Read the model definition and answer for the solid it produces. Units are mm, in the model's axes. A direction names the side the tool comes from. Coordinates: 2 decimals unless noted, no trailing zeros. Order: outer loops, then holes, each group sorted by start corner. A loop starts at its lowest first (then second) coordinate and runs counter-clockwise, first axis right, second up. Notation, with made-up numbers: (-4, 15) - (38, 15) arc R18 cw to (38, 42) - close; hole circle Ø9 at (-0.75, 27.5). An arc over 180 degrees is marked (long way). Write item = value, one per line.
from build123d import *

# Parameters (mm, degrees)
SKETCH1_W              = 116.84
SKETCH1_H              = 103.134084814
SKETCH1_R              = 3.15
BOSS_EXTRUDE1_DEPTH    = 5
SKETCH12_W             = 85
SKETCH12_H             = 23.975046692
BOSS_EXTRUDE15_DEPTH   = 5
SKETCH17_W             = 50
SKETCH17_H             = 50
BOSS_EXTRUDE18_DEPTH   = 6
SKETCH10_W             = 39.5
SKETCH10_H             = 39.5
BOSS_EXTRUDE19_DEPTH   = 25
SKETCH19_W             = 55
SKETCH19_H             = 55
BOSS_EXTRUDE20_DEPTH   = 11
SKETCH20_R             = 2.25
BOSS_EXTRUDE22_DEPTH   = 25
BOSS_EXTRUDE22_2_DEPTH = 25
BOSS_EXTRUDE22_3_DEPTH = 25
BOSS_EXTRUDE22_4_DEPTH = 25
SKETCH21_W             = 24.5
SKETCH21_H             = 21.5
BOSS_EXTRUDE23_DEPTH   = 4
SKETCH21_W_2           = 21.5
SKETCH21_H_2           = 24.5
BOSS_EXTRUDE23_2_DEPTH = 4
BOSS_EXTRUDE23_3_DEPTH = 4
BOSS_EXTRUDE23_4_DEPTH = 4
SKETCH25_R             = 4
BOSS_EXTRUDE24_DEPTH   = 3.25
BOSS_EXTRUDE24_2_DEPTH = 3.25
BOSS_EXTRUDE24_3_DEPTH = 3.25
BOSS_EXTRUDE24_4_DEPTH = 3.25


with BuildPart() as part:
    # Sketch1 → Boss-Extrude1 (new body)
    with BuildSketch(Plane(origin=(0, 0, 0), x_dir=(1, 0, 0), z_dir=(0, 1, 0))):
        with Locations((0, 1.415042407)):
            Rectangle(SKETCH1_W, SKETCH1_H)
        with Locations((-50.8, 46.711)):
            Circle(SKETCH1_R, mode=Mode.SUBTRACT)
        with Locations((50.8, -42.532)):
            Circle(SKETCH1_R, mode=Mode.SUBTRACT)
        with Locations((-50.8, -42.532)):
            Circle(SKETCH1_R, mode=Mode.SUBTRACT)
        with Locations((50.8, 46.711)):
            Circle(SKETCH1_R, mode=Mode.SUBTRACT)
    extrude(amount=-BOSS_EXTRUDE1_DEPTH)


with BuildPart() as body_2:
    # Sketch12 → Boss-Extrude15 (new body)
    with BuildSketch(Plane(origin=(0, 0, 0), x_dir=(1, 0, 0), z_dir=(0, 1, 0))):
        with Locations((0, 58)):
            Rectangle(SKETCH12_W, SKETCH12_H)
    extrude(amount=BOSS_EXTRUDE15_DEPTH)


with BuildPart() as body_3:
    # Sketch17 → Boss-Extrude18 (new body)
    with BuildSketch(Plane(origin=(0, 0, 0), x_dir=(1, 0, 0), z_dir=(0, 1, 0))):
        Rectangle(SKETCH17_W, SKETCH17_H)
    extrude(amount=-BOSS_EXTRUDE18_DEPTH)


with BuildPart() as body_4:
    # Sketch10 → Boss-Extrude19 (new body, symmetric)
    with BuildSketch(Plane(origin=(0, 0, 0), x_dir=(1, 0, 0), z_dir=(0, 1, 0))):
        Rectangle(SKETCH10_W, SKETCH10_H)
    extrude(amount=BOSS_EXTRUDE19_DEPTH, both=True)


with BuildPart() as body_5:
    # Sketch19 → Boss-Extrude20 (new body)
    with BuildSketch(Plane(origin=(0, 0, 0), x_dir=(1, 0, 0), z_dir=(0, 1, 0))):
        Rectangle(SKETCH19_W, SKETCH19_H)
    extrude(amount=-BOSS_EXTRUDE20_DEPTH)


with BuildPart() as part_1:
    add(part.part)

    # Combine1: cut body 2
    add(body_2.part, mode=Mode.SUBTRACT)


with BuildPart() as body_3_1:
    # Body-Move/Copy4: moved
    add(body_3.part.moved(Location((0, -6, 0))))


with BuildPart() as body_5_1:
    add(body_5.part)

    # Combine4: cut body 3
    add(body_3_1.part, mode=Mode.SUBTRACT)

    # Combine7: union part
    add(part_1.part)

    # Combine8: cut body 4
    add(body_4.part, mode=Mode.SUBTRACT)


with BuildPart() as body_2_2:
    # Sketch20 → Boss-Extrude22 (new body, symmetric)
    with BuildSketch(Plane(origin=(0, 0, 0), x_dir=(1, 0, 0), z_dir=(0, 1, 0))):
        with Locations((27.5, 27.5)):
            Circle(SKETCH20_R)
    extrude(amount=BOSS_EXTRUDE22_DEPTH, both=True)


with BuildPart() as body_3_2:
    # Sketch20 → Boss-Extrude22 2 (new body, symmetric)
    with BuildSketch(Plane(origin=(0, 0, 0), x_dir=(1, 0, 0), z_dir=(0, 1, 0))):
        with Locations((27.5, -27.5)):
            Circle(SKETCH20_R)
    extrude(amount=BOSS_EXTRUDE22_2_DEPTH, both=True)


with BuildPart() as body_4_2:
    # Sketch20 → Boss-Extrude22 3 (new body, symmetric)
    with BuildSketch(Plane(origin=(0, 0, 0), x_dir=(1, 0, 0), z_dir=(0, 1, 0))):
        with Locations((-27.5, -27.5)):
            Circle(SKETCH20_R)
    extrude(amount=BOSS_EXTRUDE22_3_DEPTH, both=True)


with BuildPart() as body_5_2:
    # Sketch20 → Boss-Extrude22 4 (new body, symmetric)
    with BuildSketch(Plane(origin=(0, 0, 0), x_dir=(1, 0, 0), z_dir=(0, 1, 0))):
        with Locations((-27.5, 27.5)):
            Circle(SKETCH20_R)
    extrude(amount=BOSS_EXTRUDE22_4_DEPTH, both=True)


with BuildPart() as body_5_3:
    add(body_5_1.part)

    # Combine9: cut body 4 2, body 3 2, body 2 2, body 5 2
    add(body_4_2.part, mode=Mode.SUBTRACT)
    add(body_3_2.part, mode=Mode.SUBTRACT)
    add(body_2_2.part, mode=Mode.SUBTRACT)
    add(body_5_2.part, mode=Mode.SUBTRACT)


with BuildPart() as body_2_3:
    # Sketch21 → Boss-Extrude23 (new body)
    with BuildSketch(Plane(origin=(0, 0, 0), x_dir=(1, 0, 0), z_dir=(0, 1, 0))):
        with Locations((0, 31.5)):
            Rectangle(SKETCH21_W, SKETCH21_H)
    extrude(amount=-BOSS_EXTRUDE23_DEPTH)


with BuildPart() as body_3_3:
    # Sketch21 → Boss-Extrude23 2 (new body)
    with BuildSketch(Plane(origin=(0, 0, 0), x_dir=(1, 0, 0), z_dir=(0, 1, 0))):
        with Locations((31.5, 0)):
            Rectangle(SKETCH21_W_2, SKETCH21_H_2)
    extrude(amount=-BOSS_EXTRUDE23_2_DEPTH)


with BuildPart() as body_4_3:
    # Sketch21 → Boss-Extrude23 3 (new body)
    with BuildSketch(Plane(origin=(0, 0, 0), x_dir=(1, 0, 0), z_dir=(0, 1, 0))):
        with Locations((-31.5, 0)):
            Rectangle(SKETCH21_W_2, SKETCH21_H_2)
    extrude(amount=-BOSS_EXTRUDE23_3_DEPTH)


with BuildPart() as body_5_3_1:
    # Sketch21 → Boss-Extrude23 4 (new body)
    with BuildSketch(Plane(origin=(0, 0, 0), x_dir=(1, 0, 0), z_dir=(0, 1, 0))):
        with Locations((0, -31.5)):
            Rectangle(SKETCH21_W, SKETCH21_H)
    extrude(amount=-BOSS_EXTRUDE23_4_DEPTH)


with BuildPart() as body_5_4:
    add(body_5_3.part)

    # Combine10: cut body 3 3, body 2 3, body 5 3, body 4 3
    add(body_3_3.part, mode=Mode.SUBTRACT)
    add(body_2_3.part, mode=Mode.SUBTRACT)
    add(body_5_3_1.part, mode=Mode.SUBTRACT)
    add(body_4_3.part, mode=Mode.SUBTRACT)


with BuildPart() as body_2_4:
    # Sketch25 → Boss-Extrude24 (new body)
    with BuildSketch(Plane(origin=(0, 0, 0), x_dir=(1, 0, 0), z_dir=(0, 1, 0))):
        with Locations((27.5, 27.5)):
            Circle(SKETCH25_R)
    extrude(amount=-BOSS_EXTRUDE24_DEPTH)


with BuildPart() as body_3_4:
    # Sketch25 → Boss-Extrude24 2 (new body)
    with BuildSketch(Plane(origin=(0, 0, 0), x_dir=(1, 0, 0), z_dir=(0, 1, 0))):
        with Locations((-27.5, 27.5)):
            Circle(SKETCH25_R)
    extrude(amount=-BOSS_EXTRUDE24_2_DEPTH)


with BuildPart() as body_4_4:
    # Sketch25 → Boss-Extrude24 3 (new body)
    with BuildSketch(Plane(origin=(0, 0, 0), x_dir=(1, 0, 0), z_dir=(0, 1, 0))):
        with Locations((-27.5, -27.5)):
            Circle(SKETCH25_R)
    extrude(amount=-BOSS_EXTRUDE24_3_DEPTH)


with BuildPart() as body_5_4_1:
    # Sketch25 → Boss-Extrude24 4 (new body)
    with BuildSketch(Plane(origin=(0, 0, 0), x_dir=(1, 0, 0), z_dir=(0, 1, 0))):
        with Locations((27.5, -27.5)):
            Circle(SKETCH25_R)
    extrude(amount=-BOSS_EXTRUDE24_4_DEPTH)


with BuildPart() as body_5_5:
    add(body_5_4.part)

    # Combine11: cut body 4 4, body 3 4, body 2 4, body 5 4
    add(body_4_4.part, mode=Mode.SUBTRACT)
    add(body_3_4.part, mode=Mode.SUBTRACT)
    add(body_2_4.part, mode=Mode.SUBTRACT)
    add(body_5_4_1.part, mode=Mode.SUBTRACT)


solid = body_5_5.part
1) For faces 1 (the face through (24.55, -1.6, 24.8)), 2 (the face through (0, -8, 25)), 3 (the face through (-19.75, -3, 0)), determine the directions among +Z, -Z, +X, -X, +Y, -Y from which every point of the face is accessible in a straight line to the end or side of a thin tool.
Returned:
face_1 = +Y
face_2 = -Y
face_3 = +Y, -Y
2) The part is cut by section B-B (x = 50.8). Determine the outline of the cut face in (y, z).
Returned:
outline = (-5, -52.98) - (0, -52.98) - (0, -49.86) - (-5, -49.86) - close; (-5, -43.56) - (0, -43.56) - (0, 39.38) - (-5, 39.38) - close; (-5, 45.68) - (0, 45.68) - (0, 50.15) - (-5, 50.15) - close
3) Flat-ended cylindrical pins translate along their axes: pin 1 Ø6.5 at (x, y) = (3.5, -8.5) entering from -Z; pin 2 Ø5 at (x, y) = (-3, -7) entering from +Z; pin 3 Ø1 at (y, z) = (-7.5, 28.5) entering from +X; pin 4 Ø5.5 at (x, y) = (7.5, -9) entering from +Z. Find the tip coordinate at first contact, or state that the pin passes through.
Returned:
pin_1 = -27.5
pin_2 = 50.15
pin_3 = through
pin_4 = 27.5
4) The part is cut by section D-D (y = -7.5). Determine the outline of the cut face in (x, z), and give its area (3 significant figures).
Returned:
outline = (-27.5, -25.25) arc R2.25 cw to (-25.25, -27.5) - (25.25, -27.5) arc R2.25 cw to (27.5, -25.25) - (27.5, 25.25) arc R2.25 cw to (25.25, 27.5) - (-25.25, 27.5) arc R2.25 cw to (-27.5, 25.25) - close; hole (-25, -25) - (25, -25) - (25, 25) - (-25, 25) - close
area = 509 mm^2
5) Determine the mould class of faces 4 (the face through (0, -8, -27.5)), 5 (the face through (-27.5, -8, 0)), 6 (the face through (0, -2, 42.25)) for opening direction Z: pulls with the +Z half, pulls with the -Z half, needs draft (parallel to the pull), parting line crosses it, or undercut.
Returned:
face_4 = pulls with the -Z half
face_5 = needs draft
face_6 = undercut
6) The part is cut by section C-C (x = 36). Determine the outline of the cut face in (y, z), and give its area (3 significant figures).
Returned:
outline = (-5, -52.98) - (0, -52.98) - (0, -12.25) - (-4, -12.25) - (-4, 12.25) - (0, 12.25) - (0, 50.15) - (-5, 50.15) - close
area = 418 mm^2
7) The part is cut by section A-A (z = -14). Determine the outline of the cut face in (x, y), and give its area (3 significant figures).
Returned:
outline = (-58.42, -5) - (-27.5, -5) - (-27.5, -11) - (-25, -11) - (-25, -6) - (-19.75, -6) - (-19.75, 0) - (-58.42, 0) - close; (19.75, -6) - (25, -6) - (25, -11) - (27.5, -11) - (27.5, -5) - (58.42, -5) - (58.42, 0) - (19.75, 0) - close
area = 427 mm^2
8) Straight lines are drawn through the part: line 1 along X through (y, z) = (-2.3, 27.5); line 2 along Z through (x, y) = (50.8, -3.7); line 3 along X through (y, z) = (-4.25, 5.5). For each, find the intervals that lie inside material, in ascending order. Write a range as from..to.
Returned:
line_1 = -58.42..-31.5, -23.5..-12.25, 12.25..23.5, 31.5..58.42
line_2 = -52.98..-49.86, -43.56..39.38, 45.68..50.15
line_3 = -58.42..-19.75, 19.75..58.42
